Could you check a few things on this drawing? It's one solid part, dimensions in mm from its lowest x, y, z. A direction names the side the tool comes from. Round coordinates to 2 decimals unless told otherwise and drop trailing zeros. Write each loop counter-clockwise with the first axis right and the second up, starting at its lowest first coordinate (ties: lowest second). Pieces come first, ordered by that corner, then holes. Notation, with made-up numbers: (-2.5, -20) -> (22.5, -20) arc R9 ccw to (22.5, -3) -> close; hole circle Ø10 at (81.25, 32). An arc over 180 degrees is marked (long way). Answer in a Markdown table with one row per item.
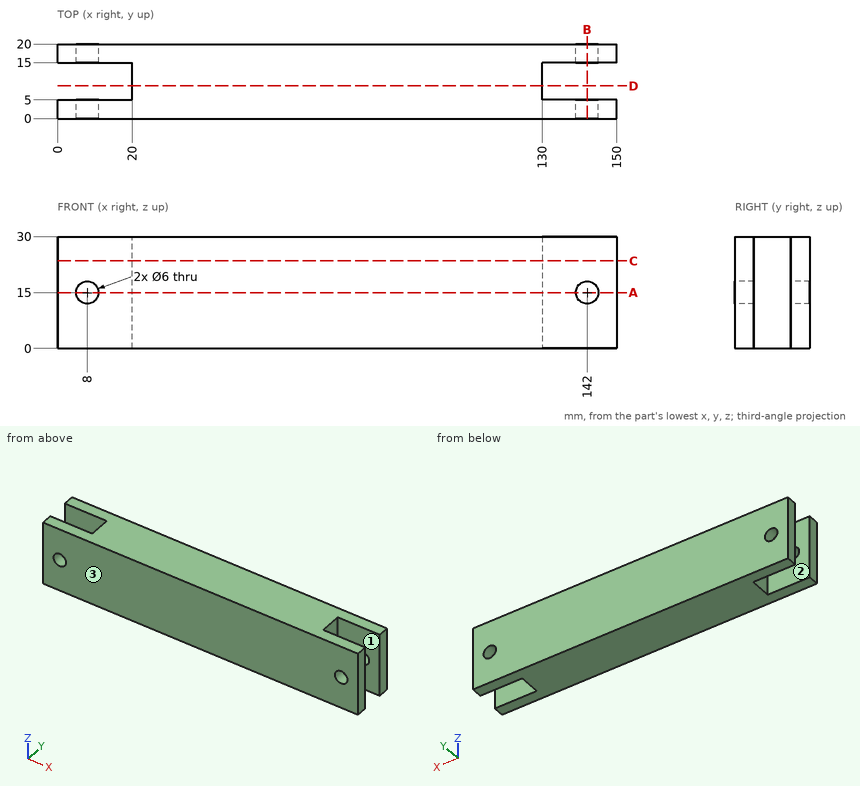
1) Imagine slicing it at C-C, the plane z = 23.5. Please give me the cut outline in (x, y).
Findings:
| item | result |
|---|---|
| outline | (0, 0) -> (150, 0) -> (150, 5) -> (130, 5) -> (130, 15) -> (150, 15) -> (150, 20) -> (0, 20) -> (0, 15) -> (20, 15) -> (20, 5) -> (0, 5) -> close |
2) For pin 1 (3 mm diameter, centred on y = 12, z = 8.5, fed in from +X); pin 2 (5.5 mm diameter, centred on x = 142, z = 15, fed in from +Y); pin 3 (8 mm diameter, centred on y = 8.5, z = 12, fed in from -X), each with a flat end and sliding along its axis, tell me the tip position at first contact or that it passes through.
Findings:
| item | result |
|---|---|
| pin 1 | stops at x = 130 |
| pin 2 | passes through |
| pin 3 | stops at x = 0 |
3) Imagine slicing it at A-A, the plane z = 15. Please give me the cut outline in (x, y).
Findings:
| item | result |
|---|---|
| outline | (0, 0) -> (5, 0) -> (5, 5) -> (0, 5) -> close; (0, 15) -> (5, 15) -> (5, 20) -> (0, 20) -> close; (11, 0) -> (139, 0) -> (139, 5) -> (130, 5) -> (130, 15) -> (139, 15) -> (139, 20) -> (11, 20) -> (11, 15) -> (20, 15) -> (20, 5) -> (11, 5) -> close; (145, 0) -> (150, 0) -> (150, 5) -> (145, 5) -> close; (145, 15) -> (150, 15) -> (150, 20) -> (145, 20) -> close |
4) For the marked faces 1, 2 and 3, which set-ups out of +Z, -Z, +X, -X, +Y, -Y let a thin tool reach every point of the face, with its end or its side?
Findings:
| item | result |
|---|---|
| face 1 | +Z, -Z, +X |
| face 2 | +Z, -Z, -X |
| face 3 | +Z, -Z, +X, -X, -Y |
5) Please list where these lines run through material, in increasing order: line 1 (X direction, y = 2.8, z = 15); line 2 (Y direction, x = 10, z = 26); line 3 (Z direction, x = 142, y = 16.7).
Findings:
| item | result |
|---|---|
| line 1 | x = 0 to 5, 11 to 139, 145 to 150 |
| line 2 | y = 0 to 5, 15 to 20 |
| line 3 | z = 0 to 12, 18 to 30 |
6) Imagine slicing it at D-D, the plane y = 8.75. Please give me the cut outline in (x, z), plus the area to 3 significant figures.
Findings:
| item | result |
|---|---|
| outline | (20, 0) -> (130, 0) -> (130, 30) -> (20, 30) -> close |
| area | 3,300 mm^2 |
7) Imagine slicing it at B-B, the plane x = 142. Please give me the cut outline in (y, z), plus the area to 3 significant figures.
Findings:
| item | result |
|---|---|
| outline | (0, 0) -> (5, 0) -> (5, 12) -> (0, 12) -> close; (0, 18) -> (5, 18) -> (5, 30) -> (0, 30) -> close; (15, 0) -> (20, 0) -> (20, 12) -> (15, 12) -> close; (15, 18) -> (20, 18) -> (20, 30) -> (15, 30) -> close |
| area | 240 mm^2 |
